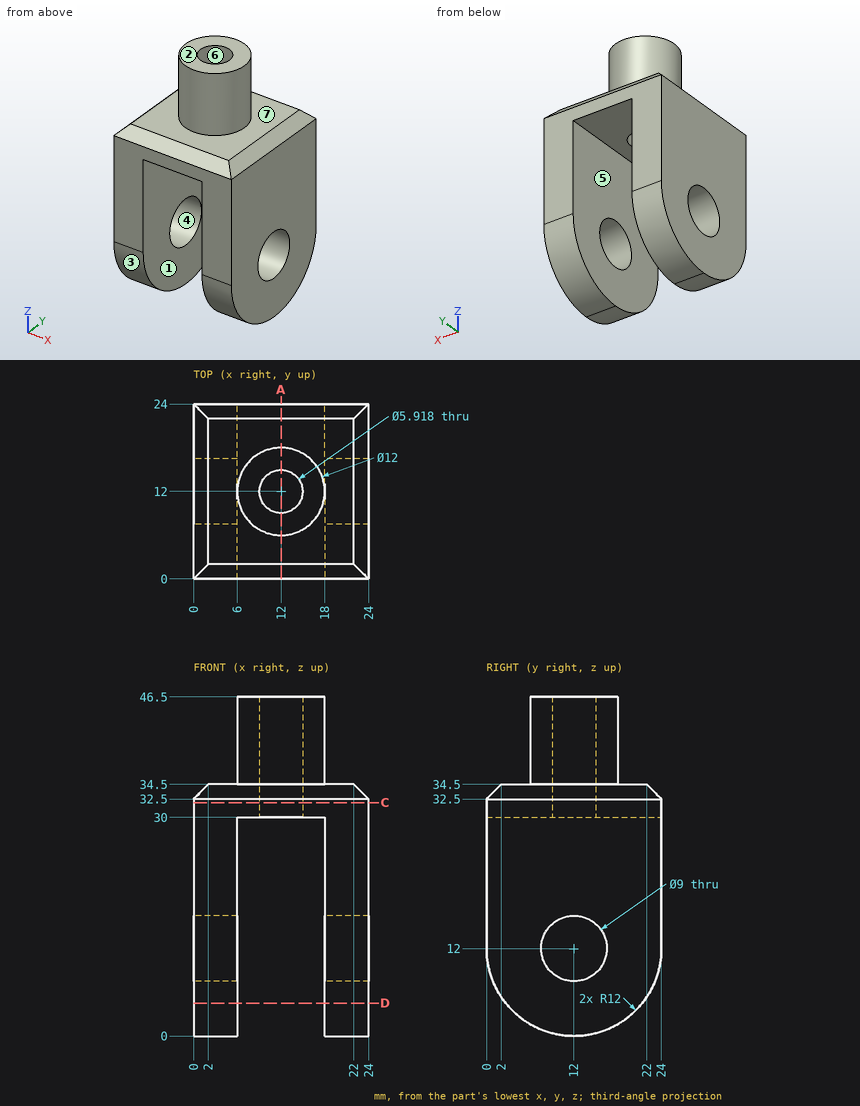
Verification items for this drawing (mm, ordinates from the low corner). A direction names the side the tool comes from. Coordinates: 2 decimals unless noted, no trailing zeros. Order: outer loops, then holes, each group sorted by start corner. A loop starts at its lowest first (then second) coordinate and runs counter-clockwise, first axis right, second up. Notation, with made-up numbers: (12, 49) - (38, 49) arc R28 cw to (38, 70) - close; hole circle Ø8 at (18.25, 1.5). An arc over 180 degrees is marked (long way). Answer in a Markdown table with one row per item. Add a question column.
1. Section check D-D (z = 4.5). Enter the section's corners in (x, y).
2. Material ranges on L1, parallel to Z at x = 2, y = 12; L2, parallel to X at y = 20.5, z = 27; L3, parallel to Y at x = 12, z = 42.5, recorded low to high. Write a range as [from, to].
3. Section check C-C (z = 32). Enter the section's corners in (x, y).
4. Access from +Z, -Z, +X, -X, +Y, -Y to the whole of each face (thin tool, end or side, straight path). Record for the marked faces 5, 6 and 7.
5. Draft check along Z on the marked faces 1, 2, 3 and 4. Enter one of: +Z half, -Z half, draft (parallel to the pull), parting line (faces both ways), or undercut.
6. Gauge pin test, flat ends, axial feed: pin 1 Ø12 at (x, y) = (20, 2.5) entering from +Z; pin 2 Ø9.5 at (x, y) = (12, 15) entering from -Z. Record the tip position at first contact, or that the pin passes through.
7. Section check A-A (x = 12). Enter the section's corners in (y, z).
Data:
| question | item | result |
|---|---|---|
| 1 | outline | (0, 2.63) - (6, 2.63) - (6, 21.37) - (0, 21.37) - close; (18, 2.63) - (24, 2.63) - (24, 21.37) - (18, 21.37) - close |
| 2 | L1 | z = [0, 7.5], [16.5, 34.5] |
| 2 | L2 | x = [0, 6], [18, 24] |
| 2 | L3 | y = [6, 9.04], [14.96, 18] |
| 3 | outline | (0, 0) - (24, 0) - (24, 24) - (0, 24) - close; hole circle Ø5.92 at (12, 12) |
| 4 | face 5 | -Z, +Y, -Y |
| 4 | face 6 | +Z, -Z |
| 4 | face 7 | +Z |
| 5 | face 1 | draft |
| 5 | face 2 | +Z half |
| 5 | face 3 | -Z half |
| 5 | face 4 | undercut |
| 6 | pin 1 | stops at z = 34.5 |
| 6 | pin 2 | stops at z = 30 |
| 7 | outline | (0, 30) - (9.04, 30) - (9.04, 46.5) - (6, 46.5) - (6, 34.5) - (2, 34.5) - (0, 32.5) - close; (14.96, 30) - (24, 30) - (24, 32.5) - (22, 34.5) - (18, 34.5) - (18, 46.5) - (14.96, 46.5) - close |
